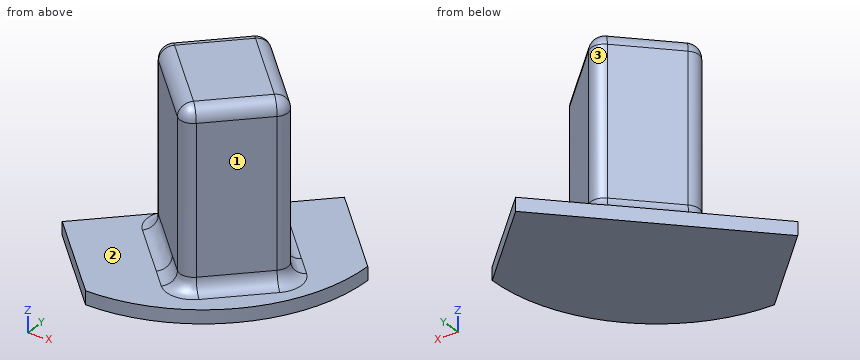
Autodesk Inventor part; units mm, degrees
ref_plane "YZ Plane" through (0, 0, 0) normal (1, 0, 0) x (0, 1, 0)
ref_plane "XZ Plane" through (0, 0, 0) normal (0, 1, 0) x (-1, 0, 0)
ref_plane "XY Plane" through (0, 0, 0) normal (0, 0, 1) x (1, 0, 0)
ref_plane "Plan de construction1" through (0, 0, 0) normal (0, 0, 1) x (1, 0, 0)
sketch "Esquisse1" plane through (0, 0, 0) normal (0, 0, 1) x (1, 0, 0)
  line L0 (12.600402, 13.369459) -> (-37.128252, -35.732002)
  line L1 (-42.505343, -6.84222) -> (-16.505712, -33.167478)
  line L2 (8.432313, -8.537922) -> (-17.567318, 17.787336)
  line L3 (-17.567318, 17.787336) -> (-42.505343, -6.84222)
  spline S0 degree 3 poles (-30.559567, -18.937609) (-29.251135, -19.178539) (-27.810091, -19.446017) (-24.924717, -19.685136) (-23.47934, -19.643963) (-21.695605, -19.298823) (-21.177712, -19.167045) (-20.168818, -18.825553) (-19.677941, -18.615468) (-18.84768, -18.187738) (-18.426343, -17.934552) (-17.631099, -17.362687) (-17.257309, -17.043846) (-16.938864, -16.72934) knots 0 0 0 0 0.39912855 0.39912855 0.7982571 0.7982571 0.94417416 0.94417416 1.09009122 1.09009122 1.22436299 1.22436299 1.35863477 1.35863477 1.35863477 1.35863477
  spline S1 degree 3 poles (-7.999161, -7.900216) (-7.680716, -7.58571) (-7.357248, -7.215917) (-6.77553, -6.427852) (-6.517119, -6.009699) (-6.079089, -5.184826) (-5.862912, -4.696602) (-5.508889, -3.692036) (-5.370676, -3.175823) (-5.003363, -1.396522) (-4.944203, 0.048231) (-5.147393, 2.936358) (-5.396916, 4.380619) (-5.621542, 5.691948) knots 3.77145385 3.77145385 3.77145385 3.77145385 3.90572563 3.90572563 4.0399974 4.0399974 4.18591446 4.18591446 4.33183152 4.33183152 4.73096007 4.73096007 5.13008862 5.13008862 5.13008862 5.13008862
  line L4 (-16.938864, -16.72934) -> (-7.999161, -7.900216)
  line L5 (-17.567318, 17.787336) -> (-5.621542, 5.691948)
  line L6 (-17.567318, 17.787336) -> (-42.505343, -6.84222)
  line L7 (-42.505343, -6.84222) -> (-30.559567, -18.937609)
  arc A0 (-30.559567, -18.937609) -> (-5.621542, 5.691948) centre (-30.176225, 5.614205) ccw
  point P0 (0, 0)
extrude "Extrusion1" add sketch "Esquisse1" along normal blind 2 contours A0 L0 L1 L3 L2 | A0 L0
sketch "Esquisse2" plane through (0, 0, 2) normal (0, 0, 1) x (1, 0, 0)
  line L0 (37.657428, -63.069018) -> (-69.549529, 45.480633)
  line L1 (37.657428, -63.069018) -> (-69.549529, 45.480633)
  line L2 (-29.434692, -3.955721) -> (-33.278207, -0.064069)
  line L3 (-33.278207, -0.064069) -> (-23.285586, 9.804949)
  line L4 (-23.285586, 9.804949) -> (-19.442072, 5.913297)
  line L5 (-24.775557, -8.673208) -> (-20.790583, -12.708092)
  line L6 (-20.790583, -12.708092) -> (-10.797962, -2.839074)
  line L7 (-10.797962, -2.839074) -> (-14.782937, 1.195809)
  line L8 (-24.775557, -8.673208) -> (-29.434692, -3.955721)
  line L9 (-19.442072, 5.913297) -> (-14.782937, 1.195809)
  point P0 (0, 0)
  point P1 (-20.366346, -4.318536)
extrude "Extrusion2" add sketch "Esquisse2" along normal blind 10
sketch "Esquisse6" plane through (-23.285586, 9.804949, 12) normal (0.7114935, 0.7026927, 0) x (0, 0, -1)
  line L0 (0, 0) -> (-15.824808, 0)
  line L1 (-15.824808, 0) -> (-15.824808, -17.771102)
  line L2 (-15.824808, -17.771102) -> (0, -17.771102)
  line L3 (0, -17.771102) -> (0, 0)
  point P0 (12, -23.338769)
  point P1 (0, -17.771102)
extrude "Extrusion6" add sketch "Esquisse6" against normal up to surface (14.044571 mm away)
fillet "Congé4" radius 2 8 edges at (-33.2782, -0.0641, 14.9124) (-23.2856, 9.8049, 14.9124) (-20.7906, -12.7081, 14.9124) (-15.7943, -7.7736, 2) (-17.0418, 3.4829, 2) (-27.0344, -6.3861, 2) (-28.2819, 4.8704, 2) (-10.798, -2.8391, 14.9124)
fillet_without_effect "Congé6"
fillet "Congé7" radius 2 8 edges at (-11.6264, -2.8339, 27.8248) (-32.4498, -0.0692, 27.8248) (-20.7854, -11.8797, 27.8248) (-15.7943, -7.7736, 27.8248) (-23.2907, 8.9765, 27.8248) (-17.0418, 3.4829, 27.8248) (-28.2819, 4.8704, 27.8248) (-27.0344, -6.3861, 27.8248)
properties part number "palette_push"
Work out the finished part from the listing and answer in its coordinate system (mm). Face numbers are marked on the shaded views. A direction names the side the tool comes from. Coordinates: 2 decimals unless noted, no trailing zeros. Write each loop counter-clockwise with the first axis right and the second up, starting at its lowest first coordinate (ties: lowest second). Pieces come first, ordered by that corner, then holes. Notation, with made-up numbers: M 17.25,54.25 L 63.25,54.25 A10 ccw 63.25,66.25 Z; hole C 2.25,42.5 d5. An arc over 180 degrees is marked long. Write item = value, one per line.
1. The part is cut by section B-B (x = -38). Determine the outline of the cut face in (y, z).
Solution:
outline = M -11.4,0 L -2.39,0 L -2.39,2 L -11.4,2 Z
2. The part is cut by section C-C (y = -15). Determine the outline of the cut face in (x, z).
Solution:
outline = M -34.45,0 L -16.83,0 L -16.83,2 L -34.45,2 Z
3. Flat-ended cylindrical pins translate along their axes: pin 1 (2 mm diameter, centred on x = -15.5, z = 16.5, fed in from -Y); pin 2 (6 mm diameter, centred on y = 7.5, z = 21.5, fed in from +X); pin 3 (4 mm diameter, centred on y = 9.5, z = 13.5, fed in from +X); pin 4 (18.5 mm diameter, centred on x = -26.5, y = -9, fed in from +Z). Find the tip coordinate at first contact, or state that the pin passes through.
Solution:
pin_1 = -8.47
pin_2 = -18.05
pin_3 = -21.01
pin_4 = 27.82
4. For the marked faces 1, 2 and 3, determine the directions among +Z, -Z, +X, -X, +Y, -Y from which every point of the face is accessible in a straight line to the end or side of a thin tool.
Solution:
face_1 = +Z, +X, -Y
face_2 = +Z
face_3 = +Z, +Y
5. Straight lines are drawn through the part: line 1 (Z direction, x = -9.5, y = -1); line 2 (X direction, y = -4.5, z = 23); line 3 (Z direction, x = -14.5, y = -7). For each, find the intervals that lie inside material, in ascending order. Write a range as from..to.
Solution:
line_1 = 0..2
line_2 = -28.9..-12.48
line_3 = 0..2.86
6. The part is cut by section A-A (z = 25.25). Determine the outline of the cut face in (x, y).
Solution:
outline = M -31.87,-1.49 L -22.2,-11.29 A2 ccw -19.37,-11.3 L -12.22,-4.24 A2 ccw -12.2,-1.42 L -21.88,8.38 A2 ccw -24.71,8.4 L -31.86,1.34 A2 ccw Z
